from build123d import *
from build123d.topology import SkipClean

# Parameters (mm, degrees)
SKETCH1_W           = 80
SKETCH1_H           = 20
BOSS_EXTRUDE1_DEPTH = 10
SKETCH2_R           = 3.5
CUT_EXTRUDE1_DEPTH  = 10
SKETCH3_R           = 3.5
BOSS_EXTRUDE2_DEPTH = 14
FILLET1_R           = 10
FILLET2_R           = 1
SKETCH4_W           = 80
SKETCH4_H           = 26
BOSS_EXTRUDE3_DEPTH = 10
FILLET6_R           = 1
SKETCH5_R           = 2
SKETCH5_R_2         = 4
CUT_EXTRUDE2_DEPTH  = 10


with BuildPart() as part:
    # Sketch1 → Boss-Extrude1 (new body)
    with BuildSketch(Plane(origin=(0, 0, 0), x_dir=(1, 0, 0), z_dir=(0, 1, 0))):
        Rectangle(SKETCH1_W, SKETCH1_H)
        with BuildLine():
            Line((-40, -10), (-40, 10))
            ThreePointArc((-40, 10), (-50, 0), (-40, -10))
        make_face()
        with BuildLine():
            ThreePointArc((40, 10), (50, 0), (40, -10))
            Line((40, -10), (40, 10))
        make_face()
    extrude(amount=BOSS_EXTRUDE1_DEPTH)

    # Sketch2 → Cut-Extrude1 (cut)
    with BuildSketch(Plane(origin=(0, 10, 0), x_dir=(1, 0, 0), z_dir=(0, 1, 0))):
        with Locations(Location((-37.125, 0, 0), (0, 0, 270))):
            Circle(SKETCH2_R)
        with Locations(Location((37.125, 0, 0), (0, 0, 270))):
            Circle(SKETCH2_R)
    extrude(amount=-CUT_EXTRUDE1_DEPTH, mode=Mode.SUBTRACT)

    # Sketch3 → Boss-Extrude2 (add)
    with SkipClean():  # the faces are left unmerged after this step: merging them gives an invalid solid
        with BuildSketch(Plane(origin=(0, 10, 0), x_dir=(1, 0, 0), z_dir=(0, 1, 0))):
            with BuildLine():
                Line((-30.726539984, 10), (-40, 10))
                ThreePointArc((-40, 10), (-50, 0), (-40, -10))
                Line((-40, -10), (-30.726539984, -10))
                Line((-30.726539984, -10), (-30.726539984, 10))
            make_face()
            with Locations((-37.125, 0)):
                Circle(SKETCH3_R, mode=Mode.SUBTRACT)
        boss_extrude2 = extrude(amount=BOSS_EXTRUDE2_DEPTH)
    add(part.part.scale(1), mode=Mode.REPLACE)  # the faces are merged on a copy

    # Mirror1: Boss-Extrude2 across plane
    with SkipClean():  # the faces are left unmerged after this step: merging them gives an invalid solid
        add(boss_extrude2.mirror(Plane(origin=(0, 0, 0), x_dir=(0, 0, 1), z_dir=(1, 0, 0))))

    # Fillet1
    fillet1_edges = [part.edges().sort_by_distance(p)[0] for p in [
        (30.726539984, 10, 0),
        (-30.726539984, 10, 0),
    ]]
    fillet(fillet1_edges, radius=FILLET1_R)

    # Fillet2
    fillet2_edges = [part.edges().sort_by_distance(p)[0] for p in [
        (-30.726539984, 22, -10),
        (-30.726539984, 24, 0),
        (-30.726539984, 22, 10),
        (-35.363269992, 24, -10),
        (-50, 24, 0),
        (-35.363269992, 24, 10),
        (35.363269992, 24, -10),
        (30.726539984, 22, -10),
        (35.363269992, 24, 10),
        (30.726539984, 22, 10),
        (50, 24, 0),
        (30.726539984, 24, 0),
        (0, 10, 10),
        (0, 10, -10),
        (27.797607796, 12.928932188, 10),
        (27.797607796, 12.928932188, -10),
        (-27.797607796, 12.928932188, 10),
        (-27.797607796, 12.928932188, -10),
    ]]
    fillet(fillet2_edges, radius=FILLET2_R)

    # Sketch4 → Boss-Extrude3 (add)
    with SkipClean():  # the faces are left unmerged after this step: merging them gives an invalid solid
        with BuildSketch(Plane(origin=(0, 0, 0), x_dir=(1, 0, 0), z_dir=(0, 1, 0))):
            with Locations((0, 23)):
                Rectangle(SKETCH4_W, SKETCH4_H)
        extrude(amount=BOSS_EXTRUDE3_DEPTH)

    # Fillet6
    # the kernel refuses this fillet: 1 mm, written as the material it adds along each edge
    with BuildSketch(Plane(origin=(-40, 10, -10), x_dir=(-0.9989642624898896, -1.4787641666586187e-15, 0.04550167324429737), z_dir=(0, -1, 0)), Plane(origin=(40, 0, -10), x_dir=(0.9989642624898897, 0, 0.04550167324429667), z_dir=(0, 1, 0))) as fillet6_piece_1:
        with BuildLine():
            CenterArc((0.955535138, 0.998964262), FILLET6_R, 182.607954285, 84.78409143)
            Line((-0.043429124, 0.953462589), (0, 0))
            ThreePointArc((0, 0), (0.455016732, 0.010357375), (0.910033465, 0))
        make_face()
    extrude(amount=10)
    # the kernel refuses this fillet: 1 mm, written as the material it takes off along each edge
    with BuildSketch(Plane(origin=(-40, -2.5, -36), x_dir=(0, 0, 1), z_dir=(0, 1, 0))) as fillet6_2_piece_1:
        with BuildLine():
            CenterArc((FILLET6_R, FILLET6_R), FILLET6_R, 180, 90)
            Line((0, FILLET6_R), (0, 0))
            Line((0, 0), (FILLET6_R, 0))
        make_face()
    extrude(amount=15, mode=Mode.SUBTRACT)
    with BuildSketch(Plane(origin=(40, -2.5, -36), x_dir=(0, 0, 1), z_dir=(0, 1, 0))) as fillet6_2_piece_2:
        with BuildLine():
            CenterArc((FILLET6_R, -FILLET6_R), FILLET6_R, 90, 90)
            Line((0, -FILLET6_R), (0, 0))
            Line((0, 0), (FILLET6_R, 0))
        make_face()
    extrude(amount=15, mode=Mode.SUBTRACT)

    # Sketch5 → Cut-Extrude2 (cut)
    with BuildSketch(Plane(origin=(0, 10, 0), x_dir=(1, 0, 0), z_dir=(0, 1, 0))):
        with Locations(Location((-9.65455784, 22, 0), (0, 0, 270))):
            Circle(SKETCH5_R)
        with Locations(Location((-17.65455784, 22, 0), (0, 0, 270))):
            Circle(SKETCH5_R_2)
        with Locations(Location((-17.65455784, 14, 0), (0, 0, 270))):
            Circle(SKETCH5_R)
        with Locations(Location((-25.65455784, 22, 0), (0, 0, 270))):
            Circle(SKETCH5_R)
        with Locations(Location((-17.65455784, 30, 0), (0, 0, 270))):
            Circle(SKETCH5_R)
        with Locations(Location((-1.65455784, 30, 0), (0, 0, 270))):
            Circle(SKETCH5_R)
        with Locations(Location((6.34544216, 22, 0), (0, 0, 270))):
            Circle(SKETCH5_R)
        with Locations(Location((-1.65455784, 14, 0), (0, 0, 270))):
            Circle(SKETCH5_R)
        with Locations(Location((-1.65455784, 22, 0), (0, 0, 270))):
            Circle(SKETCH5_R_2)
        with Locations(Location((22.34544216, 22, 0), (0, 0, 270))):
            Circle(SKETCH5_R)
        with Locations(Location((14.34544216, 14, 0), (0, 0, 270))):
            Circle(SKETCH5_R)
        with Locations(Location((14.34544216, 30, 0), (0, 0, 270))):
            Circle(SKETCH5_R)
        with Locations(Location((14.34544216, 22, 0), (0, 0, 270))):
            Circle(SKETCH5_R_2)
    extrude(amount=-CUT_EXTRUDE2_DEPTH, mode=Mode.SUBTRACT)


solid = part.part
CAD build for the part. Positions are in the model's coordinates, mm. A direction names the side the tool comes from. Give positions to 0.01 mm unless a question says otherwise; leave off trailing zeros. Loops run counter-clockwise (first coordinate to the right, second up) from the corner with the lowest first, then second, coordinate; pieces in that order, holes last. Notation, with made-up numbers: M 56,4.5 L 68,4.5 A23 ccw 68,41.5 Z; hole C 79,16 d9. An arc over 180 degrees is marked long. Write each question's results on one line, items separated by ' | '.
Q1. Which spindle directions (+Z, -Z, +X, -X, +Y, -Y) get a long thin tool onto all of the face, cutting with end or side? Do faces 1 (the face through (-30.727, 21, 0)), 2 (the face through (-1, 5, -36)), 3 (the face through (-1.2, 10, -26.4)). Say none if no direction does.
Geometry check:
face 1: +Z, -Z, +Y | face 2: -Z, +X, -X, +Y, -Y | face 3: -Z, +X, -X, +Y
Q2. Band-saw the part on A-A on z = -14. Write the cut outline in (x, y), and give its area (3 significant figures).
Geometry check:
outline: M -40,0 L -19.65,0 L -19.65,10 L -40,10 Z; M -15.65,0 L -3.65,0 L -3.65,10 L -15.65,10 Z; M 0.35,0 L 12.35,0 L 12.35,10 L 0.35,10 Z; M 16.35,0 L 40,0 L 40,10 L 16.35,10 Z | area: 680 mm²
Q3. Mould opens along X. For faces 4 (the face through (0, 10, 0)), 5 (the face through (40.5, 24, 1.9)), 6 (the face through (-50, 11, 0)), 7 (the face through (14.946, 5.07, -28.092)) say: pulls with the +X half, pulls with the -X half, needs draft (parallel to the pull), parting line crosses it, or undercut.
Geometry check:
face 4: undercut | face 5: needs draft | face 6: pulls with the -X half | face 7: undercut
Q4. Probe probe 1 along X at (y, z) = (6, 0) (3 decimals); probe 2 along X at (y, z) = (8, -14); probe 3 along X at (y, z) = (1.25, -31). List the from-to ranges inside material, lowest first.
Geometry check:
probe 1: x = -50 to -40.625, -33.625 to 33.625, 40.625 to 50 | probe 2: x = -40 to -19.65, -15.65 to -3.65, 0.35 to 12.35, 16.35 to 40 | probe 3: x = -40 to -19.39, -15.92 to -3.39, 0.08 to 12.61, 16.08 to 40
Q5. Band-saw the part on C-C on y = 3.75. Give the number of separate pieces and of enclosed holes in the cut face, and give its area (3 significant figures).
Geometry check:
separate pieces: 1 | enclosed holes: 15 | area: 3,640 mm²
Q6. Band-saw the part on B-B on z = 0. Write the cut outline in (x, y) (3 decimals).
Geometry check:
outline: M -50,0 L -40.625,0 L -40.625,24 L -49,24 A1 ccw -50,23 Z; M -33.625,0 L 33.625,0 L 33.625,24 L 31.727,24 A1 ccw 30.727,23 L 30.727,20 A10 cw 20.727,10 L -20.727,10 A10 cw -30.727,20 L -30.727,23 A1 ccw -31.727,24 L -33.625,24 Z; M 40.625,0 L 50,0 L 50,23 A1 ccw 49,24 L 40.625,24 Z
Q7. Flat gauge pins, fed straight in: P1, Ø6, axis at x = -30.5, z = -31, coming from the +Y side; P2, Ø8, axis at y = 11, z = -20, coming from the +X side; P3, Ø3, axis at y = 14, z = -3, coming from the -X side. Where does each tip first touch, or does it go through?
Geometry check:
P1: stops at y = 10 | P2: stops at x = 40 | P3: stops at x = -49.89
